Work out the finished part from the listing and answer in its coordinate system (mm). A direction names the side the tool comes from. Give positions to 0.01 mm unless a question says otherwise; leave off trailing zeros. Loops run counter-clockwise (first coordinate to the right, second up) from the corner with the lowest first, then second, coordinate; pieces in that order, holes last. Notation, with made-up numbers: M 40.25,3 L 51.25,3 A27 cw 51.25,28 Z; hole C 48.25,-18.5 d2. An arc over 180 degrees is marked long. Use a Markdown table: item, result.
```python
from build123d import *

# Parameters (mm, degrees)
F0_W     = 159.4
F0_H     = 34.4
F0_R     = 1.425
F1_DEPTH = 4.5
F0_W_2   = 163.4
F0_H_2   = 38.4
F2_DEPTH = 1.8


with BuildPart() as f1:
    # F0 (on Front) → F1 (new body)
    with BuildSketch(Plane.XZ):
        Rectangle(F0_W, F0_H)
        with Locations((-77.7, 0)):
            Circle(F0_R, mode=Mode.SUBTRACT)
        with Locations((77.7, 0)):
            Circle(F0_R, mode=Mode.SUBTRACT)
    extrude(amount=-F1_DEPTH)

    # F0 (on Front) → F2 (join)
    with BuildSketch(Plane.XZ):
        Rectangle(F0_W_2, F0_H_2)
        Rectangle(F0_W, F0_H, mode=Mode.SUBTRACT)
    extrude(amount=-F2_DEPTH)


solid = f1.part
```
(1) A cutting plane is placed at B-B (z = 0). Write down the section's boundary in (x, y) (3 decimals).
Entries:
| item | result |
|---|---|
| outline | M -81.7,0 L -79.125,0 L -79.125,4.5 L -79.7,4.5 L -79.7,1.8 L -81.7,1.8 Z; M -76.275,0 L 76.275,0 L 76.275,4.5 L -76.275,4.5 Z; M 79.125,0 L 81.7,0 L 81.7,1.8 L 79.7,1.8 L 79.7,4.5 L 79.125,4.5 Z |
(2) A cutting plane is placed at D-D (x = -6.5). Write down the section's boundary in (y, z), and give its area (3 significant figures).
Entries:
| item | result |
|---|---|
| outline | M 0,-19.2 L 1.8,-19.2 L 1.8,-17.2 L 4.5,-17.2 L 4.5,17.2 L 1.8,17.2 L 1.8,19.2 L 0,19.2 Z |
| area | 162 mm² |
(3) A cutting plane is placed at A-A (x = 77.7). Write down the section's boundary in (y, z) (3 decimals), and give its area (3 significant figures).
Entries:
| item | result |
|---|---|
| outline | M 0,-19.2 L 1.8,-19.2 L 1.8,-17.2 L 4.5,-17.2 L 4.5,-1.425 L 0,-1.425 Z; M 0,1.425 L 4.5,1.425 L 4.5,17.2 L 1.8,17.2 L 1.8,19.2 L 0,19.2 Z |
| area | 149 mm² |
(4) Consider probe 1 along Z at (x, y) = (77.7, 1.9) (3 decimals); probe 2 along Z at (x, y) = (77.7, 1.5) (3 decimals); probe 3 along X at (y, z) = (3.2, 0.5). Determine where each line is inside the solid, lowest interval first. Write a range as [from, to].
Entries:
| item | result |
|---|---|
| probe 1 | z = [-17.2, -1.425], [1.425, 17.2] |
| probe 2 | z = [-19.2, -1.425], [1.425, 19.2] |
| probe 3 | x = [-79.7, -79.03], [-76.37, 76.37], [79.03, 79.7] |
(5) The mould has two halves that part along Z. Classify faces 4 (the cylindrical face through (76.57, 2.22, -0.87)), 5 (the flat face through (-1, 3, -17.2)), 6 (the flat face through (-1, 0, 0)), 7 (the cylindrical face through (-78.83, 2.22, -0.87)): released by +Z, released by -Z, zero draft, split by the parting line, or undercut.
Entries:
| item | result |
|---|---|
| face 4 | undercut |
| face 5 | released by -Z |
| face 6 | zero draft |
| face 7 | undercut |
(6) A cutting plane is placed at C-C (y = 2.9). Write down the section's boundary in (x, z) (3 decimals), and give its area (3 significant figures).
Entries:
| item | result |
|---|---|
| outline | M -79.7,-17.2 L 79.7,-17.2 L 79.7,17.2 L -79.7,17.2 Z; hole C -77.7,0 d2.85; hole C 77.7,0 d2.85 |
| area | 5,470 mm² |
(7) Which of the six approach directions +Z, -Z, +X, -X, +Y, -Y give full straight-line access (tool end or side, diameter ignored) to faces 1 (the flat face through (-79.7, 3, 0)), 2 (the flat face through (79.7, 3, 0)), 3 (the flat face through (-1, 3, 17.2))?
Entries:
| item | result |
|---|---|
| face 1 | +Z, -Z, -X, +Y |
| face 2 | +Z, -Z, +X, +Y |
| face 3 | +Z, +X, -X, +Y |
(8) Given P1, Ø2, axis at y = 3.5, z = 3, coming from the +X side; P2, Ø0.8, axis at x = 13, y = 2.5, coming from the +Z side; P3, Ø2, axis at y = 3, z = -8, coming from the -X side; P4, Ø2.5, axis at x = 77.7, z = 0, coming from the +Y side, each flat-ended and moving along its own axis, determine where each tip first touches the part or whether it passes through.
Entries:
| item | result |
|---|---|
| P1 | stops at x = 79.7 |
| P2 | stops at z = 17.2 |
| P3 | stops at x = -79.7 |
| P4 | passes through |
